Answer from the drawing. Dimensions are ordinates in mm from the lowest x, y and z of the part. A direction names the side the tool comes from. Give positions to 0.01 mm unless a question says otherwise; leave off trailing zeros. Loops run counter-clockwise (first coordinate to the right, second up) from the corner with the lowest first, then second, coordinate; pieces in that order, holes last.
(1) Find section B-B, the plane x = 65. Write down the section's boundary in (y, z).
(2) Find section C-C, the plane y = 15.5. Write down the section's boundary in (x, z).
(3) Find section D-D, the plane z = 118.5. Write down the section's boundary in (x, y).
(4) Find section A-A, the plane z = 135. Write down the section's boundary in (x, y).
(5) Determine the mould class of the marked faces 3, 4 and 5 for opening direction Z: pulls with the +Z half, pulls with the -Z half, needs draft (parallel to the pull), parting line crosses it, or undercut.
(6) Each of these flat-tipped pins is pushed along its axis until it touches: P1, Ø3.5, axis at x = 87.76, z = 128.94, coming from the +Y side; P2, Ø5, axis at x = 83.5, z = 72.5, coming from the +Y side. Where does it stop, or does it pass through?
(7) Straight lines are drawn through the part: probe 1 along X at (y, z) = (0.85, 45); probe 2 along X at (y, z) = (10.25, 110); probe 3 along Z at (x, y) = (83.5, 8.5). For each, find the intervals that lie inside material, in ascending order.
(8) Which of the six approach directions +Z, -Z, +X, -X, +Y, -Y give full straight-line access (tool end or side, diameter ignored) to the marked faces 1 and 2?
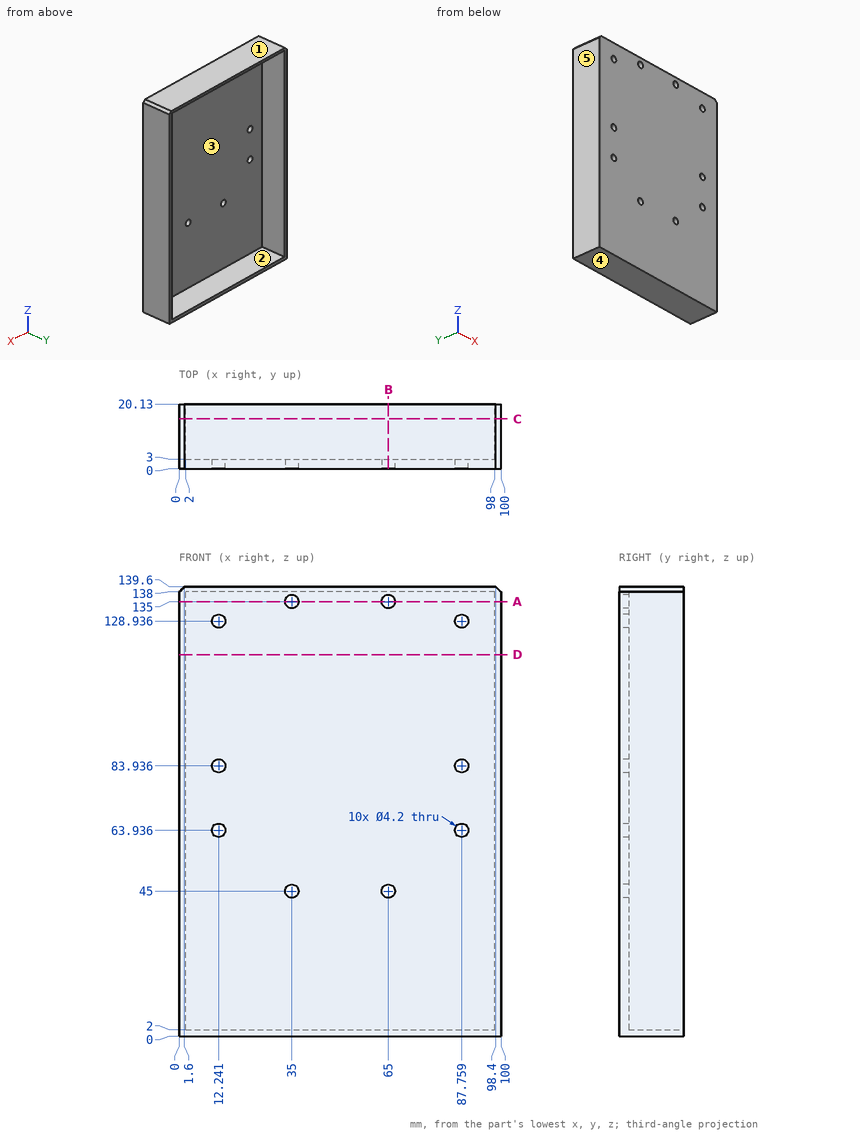
Entries:
1. outline: (0, 0) - (20.13, 0) - (20.13, 2) - (3, 2) - (3, 42.9) - (0, 42.9) - close; (0, 47.1) - (3, 47.1) - (3, 132.9) - (0, 132.9) - close; (0, 137.1) - (3, 137.1) - (3, 138) - (20.13, 138) - (20.13, 139.6) - (0, 139.6) - close
2. outline: (0, 0) - (100, 0) - (100, 138) - (98.4, 139.6) - (1.6, 139.6) - (0, 138) - close; hole (2, 2) - (98, 2) - (98, 138) - (2, 138) - close
3. outline: (0, 0) - (100, 0) - (100, 20.13) - (98, 20.13) - (98, 3) - (2, 3) - (2, 20.13) - (0, 20.13) - close
4. outline: (0, 0) - (32.9, 0) - (32.9, 3) - (2, 3) - (2, 20.13) - (0, 20.13) - close; (37.1, 0) - (62.9, 0) - (62.9, 3) - (37.1, 3) - close; (67.1, 0) - (100, 0) - (100, 20.13) - (98, 20.13) - (98, 3) - (67.1, 3) - close
5. face 3: undercut
5. face 4: pulls with the -Z half
5. face 5: needs draft
6. P1: passes through
6. P2: stops at y = 3
7. probe 1: x = 0 to 32.9, 37.1 to 62.9, 67.1 to 100
7. probe 2: x = 0 to 2, 98 to 100
7. probe 3: z = 0 to 2, 138 to 139.6
8. face 1: +Z, +X, -X, +Y, -Y
8. face 2: +Y
